```python
from build123d import *

# Parameters (mm, degrees)
F0_R     = 117.475
F1_DEPTH = 596.9
F2_W     = 355.6
F2_H     = 685.8
F3_DEPTH = 558.8


with BuildPart() as f1:
    # F0 (on Top) → F1 (new body)
    with BuildSketch(Plane.XY):
        Circle(F0_R)
    extrude(amount=F1_DEPTH)

    # F2 (on Front) → F3 (join)
    with BuildSketch(Plane.XZ):
        Polygon((208.986691, -50.8), (208.986691, 0), (208.986691, 736.6), (-248.213309, 736.6), (-248.213309, -50.8), align=None)
        with Locations((-19.613309, 342.9)):
            Rectangle(F2_W, F2_H, mode=Mode.SUBTRACT)
    extrude(amount=F3_DEPTH)


solid = f1.part
```
Verification items for the finished model (mm, model axes). A direction names the side the tool comes from. Coordinates: 2 decimals unless noted, no trailing zeros. Order: outer loops, then holes, each group sorted by start corner. A loop starts at its lowest first (then second) coordinate and runs counter-clockwise, first axis right, second up. Notation, with made-up numbers: (45, 9.25) - (86, 9.25) arc R21 cw to (86, 40.25) - close; hole circle Ø3 at (51.25, -40). An arc over 180 degrees is marked (long way). Return JSON: item names as keys, results as strings.
(1) Section check C-C, the plane y = -209.5. Record the cut outline in (x, z).
Filled sheet:
{"outline": "(-248.21, -50.8) - (208.99, -50.8) - (208.99, 736.6) - (-248.21, 736.6) - close; hole (-197.41, 0) - (158.19, 0) - (158.19, 685.8) - (-197.41, 685.8) - close"}
(2) Mould release check, pull along Z, two halves, no side actions. Record for faces 4 (the flat face through (180, 0, 348)), 5 (the flat face through (-2, 47, 0)), 6 (the cylindrical face through (-93.224, -71.482, 294.272)), 7 (the flat face through (158.187, -275, 338)): pulls with the +Z half, pulls with the -Z half, needs draft (parallel to the pull), parting line crosses it, or undercut.
Filled sheet:
{"face 4": "needs draft", "face 5": "pulls with the -Z half", "face 6": "undercut", "face 7": "undercut"}
(3) Section check B-B, the plane z = 96.5. Record the cut outline in (x, y) (3 decimals).
Filled sheet:
{"outline": "(-248.213, -558.8) - (-197.413, -558.8) - (-197.413, 0) - (-248.213, 0) - close; circle Ø234.95 at (0, 0); (158.187, -558.8) - (208.987, -558.8) - (208.987, 0) - (158.187, 0) - close"}
(4) Access from +Z, -Z, +X, -X, +Y, -Y to the whole of each face (thin tool, end or side, straight path). Record for faces 1 (the flat face through (-22, -275, 685.8)), 2 (the flat face through (180, -558.8, 348)), 3 (the flat face through (-22, -338, 0)).
Filled sheet:
{"face 1": "+Y, -Y", "face 2": "+Z, -Z, +X, -X, -Y", "face 3": "-Y"}
(5) Section check D-D, the plane x = 87.5. Record the cut outline in (y, z).
Filled sheet:
{"outline": "(-558.8, -50.8) - (0, -50.8) - (0, 0) - (78.38, 0) - (78.38, 596.9) - (-78.38, 596.9) - (-78.38, 0) - (-558.8, 0) - close; (-558.8, 685.8) - (0, 685.8) - (0, 736.6) - (-558.8, 736.6) - close"}
(6) Section check A-A, the plane x = 0. Record the cut outline in (y, z) (3 decimals).
Filled sheet:
{"outline": "(-558.8, -50.8) - (0, -50.8) - (0, 0) - (117.475, 0) - (117.475, 596.9) - (-117.475, 596.9) - (-117.475, 0) - (-558.8, 0) - close; (-558.8, 685.8) - (0, 685.8) - (0, 736.6) - (-558.8, 736.6) - close"}
(7) Thickness scan on line 1 along X through (y, z) = (-148, 391); line 2 along Z through (x, y) = (-152, -254); line 3 along Z through (x, y) = (31.5, -77.5). Record the ranges inside material, lowest first.
Filled sheet:
{"line 1": "x = -248.21 to -197.41, 158.19 to 208.99", "line 2": "z = -50.8 to 0, 685.8 to 736.6", "line 3": "z = -50.8 to 596.9, 685.8 to 736.6"}
(8) Go/stop test with flat-tipped pins: pin 1 (5 mm diameter, centred on x = 163, z = 363.5, fed in from +Y); pin 2 (10 mm diameter, centred on x = 62, z = 200.5, fed in from -Y); pin 3 (6 mm diameter, centred on x = 59, z = 437.5, fed in from +Y). Record where each tip stops, or that it passes through.
Filled sheet:
{"pin 1": "stops at y = 0", "pin 2": "stops at y = -102.72", "pin 3": "stops at y = 103.27"}
